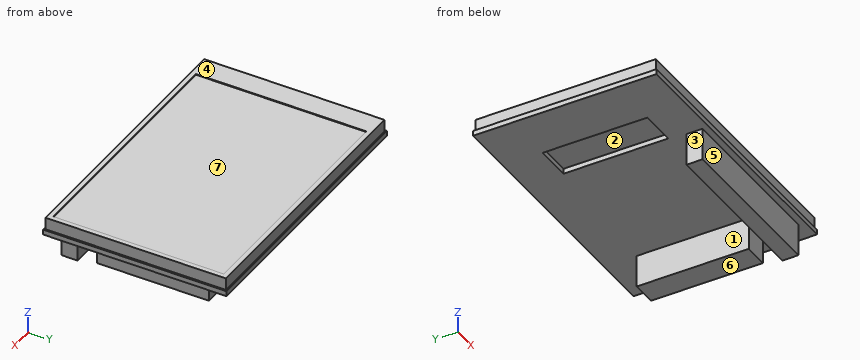
from build123d import *

# Parameters (mm, degrees)
F0_W     = 85.35
F0_H     = 56.6
F0_W_2   = 11.11
F0_H_2   = 32.25
F1_DEPTH = 1.6
F2_W     = 84.35
F2_H     = 55.6
F3_DEPTH = 3.75
F4_W     = 75.85
F4_H     = 52.6
F5_DEPTH = 0.25
F6_W     = 7.6
F6_H     = 34.6
F6_W_2   = 51
F6_H_2   = 5
F7_DEPTH = 10


with BuildPart() as f1:
    # F0 (on Top) → F1 (new body)
    with BuildSketch(Plane.XY):
        Rectangle(F0_W, F0_H)
        with Locations((-21.01, 0)):
            Rectangle(F0_W_2, F0_H_2, mode=Mode.SUBTRACT)
    extrude(amount=F1_DEPTH)

    # F2 (on face) → F3 (join)
    with BuildSketch(Plane.XY.offset(1.6)):
        Rectangle(F2_W, F2_H)
    extrude(amount=F3_DEPTH)

    # F4 (on face) → F5 (cut)
    with BuildSketch(Plane.XY.offset(5.35)):
        with Locations((2.75, 0)):
            Rectangle(F4_W, F4_H)
    extrude(amount=-F5_DEPTH, mode=Mode.SUBTRACT)

    # F6 (on face) → F7 (join)
    with BuildSketch(Plane(origin=(0, 0, 0), x_dir=(1, 0, 0), z_dir=(0, 0, -1))):
        with Locations((30.875, -1)):
            Rectangle(F6_W, F6_H)
        with Locations((10.775, 23.8)):
            Rectangle(F6_W_2, F6_H_2)
    extrude(amount=F7_DEPTH)


solid = f1.part
CAD build for the part. Positions are in the model's coordinates, mm. Face numbers are marked on the shaded views. A direction names the side the tool comes from. Coordinates: 2 decimals unless noted, no trailing zeros. Loops run counter-clockwise (first coordinate to the right, second up) from the corner with the lowest first, then second, coordinate; pieces in that order, holes last. Notation, with made-up numbers: (89, 31.5) - (114, 31.5) arc R29 ccw to (114, 67.5) - close; hole circle Ø5 at (0.25, 74). An arc over 180 degrees is marked (long way). Use one line per item in the form item = value. Start each with the question number.
1) Two-plate mould, pull along Y, no slides. Class the marked faces 5, 6 and 7: +Y half, -Y half, draft (parallel to the pull), parting line (faces both ways), or undercut.
2) Band-saw the part on D-D (x = -32.5). Give the cut face in (y, z).
3) Band-saw the part on C-C (y = -11). Give the cut face in (x, z) (3 decimals), and give its area (3 significant figures).
4) Band-saw the part on B-B (x = 21). Give the cut face in (y, z).
5) Tool access for the marked faces 1, 2, 3 and 4: list every direction of +Z, -Z, +X, -X, +Y, -Y with a clear straight run to the whole face (end or side of a thin tool).
6) Band-saw the part on A-A (z = -5). Give the cut face in (x, y) (3 decimals), and give its area (3 significant figures).
7) Flat gauge pins, fed straight in: pin 1 (6 mm diameter, centred on x = 31, z = -3.5, fed in from -Y); pin 2 (5 mm diameter, centred on x = 20, y = 21.5, fed in from -Z); pin 3 (3 mm diameter, centred on x = 8.5, z = 3.5, fed in from -Y). Where does each tip first touch, or does it go through?
8) Drill centre lines: L1, parallel to X at y = -3.5, z = 1.25 (3 decimals); L2, parallel to Z at x = -21, y = 3.5; L3, parallel to Z at x = 33.5, y = 8.5. Where is each one in solid material? Low to high. Write a range as from..to.
Check values:
q1.face_5 = -Y half
q1.face_6 = draft
q1.face_7 = undercut
q2.outline = (-28.3, 0) - (28.3, 0) - (28.3, 1.6) - (27.8, 1.6) - (27.8, 5.35) - (26.3, 5.35) - (26.3, 5.1) - (-26.3, 5.1) - (-26.3, 5.35) - (-27.8, 5.35) - (-27.8, 1.6) - (-28.3, 1.6) - close
q3.outline = (-42.675, 0) - (-26.565, 0) - (-26.565, 1.6) - (-15.455, 1.6) - (-15.455, 0) - (27.075, 0) - (27.075, -10) - (34.675, -10) - (34.675, 0) - (42.675, 0) - (42.675, 1.6) - (42.175, 1.6) - (42.175, 5.35) - (40.675, 5.35) - (40.675, 5.1) - (-35.175, 5.1) - (-35.175, 5.35) - (-42.175, 5.35) - (-42.175, 1.6) - (-42.675, 1.6) - close
q3.area = 492 mm2
q4.outline = (-28.3, 0) - (-26.3, 0) - (-26.3, -10) - (-21.3, -10) - (-21.3, 0) - (28.3, 0) - (28.3, 1.6) - (27.8, 1.6) - (27.8, 5.35) - (26.3, 5.35) - (26.3, 5.1) - (-26.3, 5.1) - (-26.3, 5.35) - (-27.8, 5.35) - (-27.8, 1.6) - (-28.3, 1.6) - close
q5.face_1 = -Z, -X, +Y
q5.face_2 = -Z
q5.face_3 = -Z, -X, +Y, -Y
q5.face_4 = +Z, +X, -X, +Y, -Y
q6.outline = (-14.725, -26.3) - (36.275, -26.3) - (36.275, -21.3) - (-14.725, -21.3) - close; (27.075, -16.3) - (34.675, -16.3) - (34.675, 18.3) - (27.075, 18.3) - close
q6.area = 518 mm2
q7.pin_1 = -26.3
q7.pin_2 = 0
q7.pin_3 = -27.8
q8.L1 = -42.675..-26.565, -15.455..42.675
q8.L2 = 1.6..5.1
q8.L3 = -10..5.1
